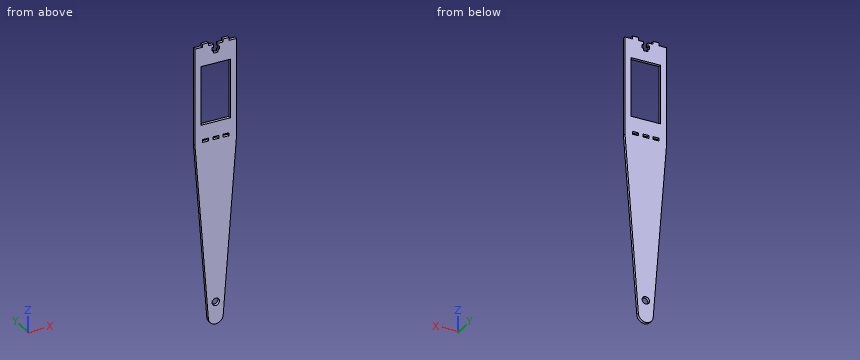
from build123d import *

# Parameters (mm, degrees)
SKETCH1_W           = 20
SKETCH1_H           = 40
SKETCH1_W_2         = 4
SKETCH1_H_2         = 2
BOSS_EXTRUDE1_DEPTH = 2
SKETCH2_R           = 2.5
BOSS_EXTRUDE2_DEPTH = 2


with BuildPart() as part:
    # Sketch1 → Boss-Extrude1 (new body)
    with BuildSketch(Plane(origin=(0, 0, 0), x_dir=(1, 0, 0), z_dir=(0, 1, 0))):
        Polygon((0, 0), (5, 0), (5, -2), (9, -2), (9, 0), (12.5, 0), (12.5, 2), (11.4, 2), (11.4, 4.3), (12.5, 4.3), (12.5, 6), (15.5, 6), (15.5, 4.3), (16.6, 4.3), (16.6, 2), (15.5, 2), (15.5, 0), (19, 0), (19, -2), (23, -2), (23, 0), (28, 0), (28, 66), (0, 66), align=None)
        with Locations((14, 33)):
            Rectangle(SKETCH1_W, SKETCH1_H, mode=Mode.SUBTRACT)
        with Locations((7, 64)):
            Rectangle(SKETCH1_W_2, SKETCH1_H_2, mode=Mode.SUBTRACT)
        with Locations((21, 64)):
            Rectangle(SKETCH1_W_2, SKETCH1_H_2, mode=Mode.SUBTRACT)
        with Locations((14, 64)):
            Rectangle(SKETCH1_W_2, SKETCH1_H_2, mode=Mode.SUBTRACT)
    extrude(amount=BOSS_EXTRUDE1_DEPTH)

    # Sketch2 → Boss-Extrude2 (add)
    with BuildSketch(Plane(origin=(0, 2, 0), x_dir=(1, 0, 0), z_dir=(0, 1, 0))):
        with BuildLine():
            Line((28, 66), (19, 186))
            ThreePointArc((19, 186), (14, 191), (9, 186))
            Line((9, 186), (0, 66))
            Line((0, 66), (28, 66))
        make_face()
        with Locations(Location((14, 176, 0), (0, 0, 270))):
            Circle(SKETCH2_R, mode=Mode.SUBTRACT)
    extrude(amount=-BOSS_EXTRUDE2_DEPTH)


solid = part.part
Here's how the part is built. I have some questions about the finished solid (model axes, mm). Round coordinates to 2 decimals unless told otherwise and drop trailing zeros. Loops run counter-clockwise (first coordinate to the right, second up) from the corner with the lowest first, then second, coordinate; pieces in that order, holes last. Notation, with made-up numbers: (16, 22.25) -> (41, 22.25) arc R26 ccw to (41, 40.25) -> close; hole circle Ø1 at (3, 33.25). An arc over 180 degrees is marked (long way). Write each question's results on one line, items separated by ' | '.
(1) If we section it at A-A, the plane z = -176: List the corners of the cut face in (x, y) for me.
Worked answers:
outline: (8.25, 0) -> (11.5, 0) -> (11.5, 2) -> (8.25, 2) -> close; (16.5, 0) -> (19.75, 0) -> (19.75, 2) -> (16.5, 2) -> close
(2) If we section it at D-D, the plane z = -146.5: List the corners of the cut face in (x, y) for me.
Worked answers:
outline: (6.04, 0) -> (21.96, 0) -> (21.96, 2) -> (6.04, 2) -> close
(3) If we section it at C-C, the plane y = 1.25: Give the number of separate pieces and of enclosed holes in the cut face, then the cut area to 3 significant figures.
Worked answers:
separate pieces: 1 | enclosed holes: 5 | area: 3,320 mm2
(4) For P1, Ø1, axis at x = 3, y = 1, coming from the +Z side; P2, Ø5, axis at x = 3, z = -164.5, coming from the -Y side; P3, Ø1.2, axis at x = 16, y = 1, coming from the -Z side, each with a flat end and sliding along its axis, tell me the tip position at first contact or that it passes through.
Worked answers:
P1: z = 0 | P2: through | P3: z = -190.8
(5) If I drill on L1, parallel to X at y = 1.45, z = -42.5; L2, parallel to Z at x = 13, y = 1.35; L3, parallel to X at y = 1.1, z = -176, over which ranges is the centre line in solid material (lowest first)?
Worked answers:
L1: 0 to 4, 24 to 28 | L2: -190.9 to -178.29, -173.71 to -65, -63 to -53, -13 to -6 | L3: 8.25 to 11.5, 16.5 to 19.75
(6) If we section it at B-B, the plane z = -48.5: List the corners of the cut face in (x, y) for me, then the cut area to 3 significant figures.
Worked answers:
outline: (0, 0) -> (4, 0) -> (4, 2) -> (0, 2) -> close; (24, 0) -> (28, 0) -> (28, 2) -> (24, 2) -> close | area: 16.0 mm2
